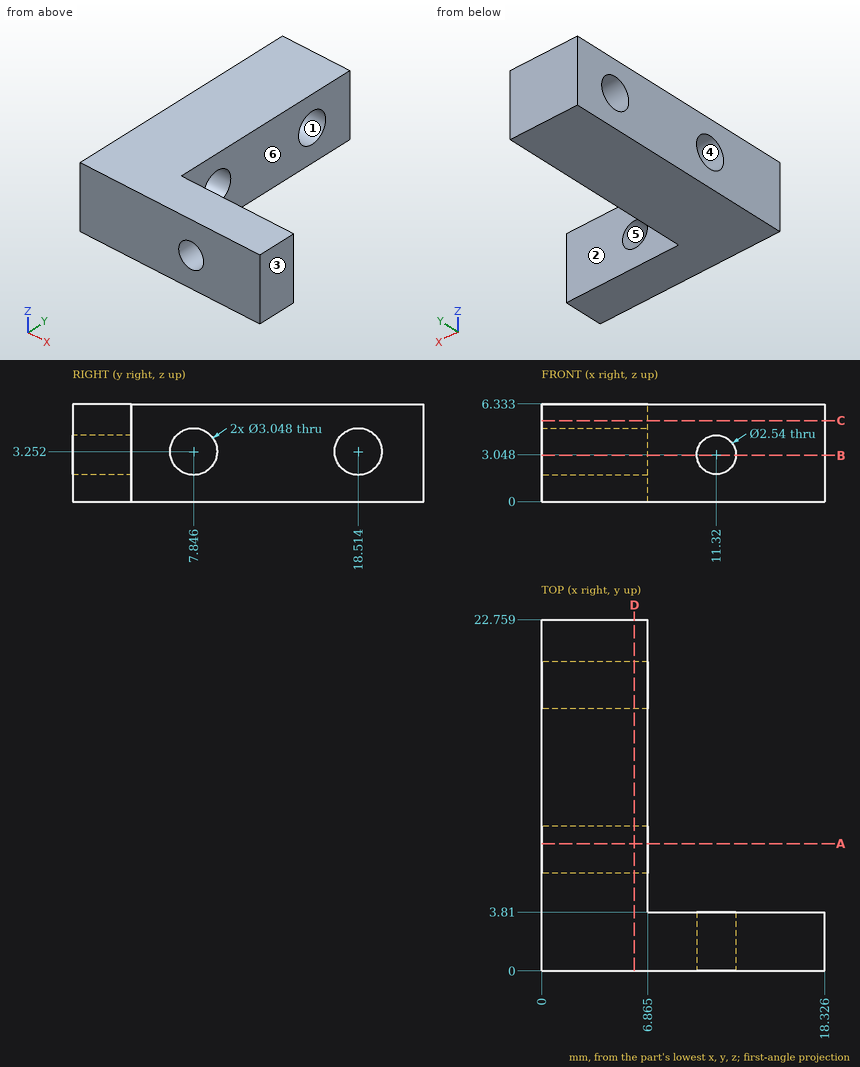
Drawing for the job (mm, zero at the part's lowest x, y, z). A direction names the side the tool comes from. Coordinates: 2 decimals unless noted, no trailing zeros. Write each loop counter-clockwise with the first axis right and the second up, starting at its lowest first coordinate (ties: lowest second). Pieces come first, ordered by that corner, then holes. Notation, with made-up numbers: (65.5, 21) -> (108.5, 21) arc R15 ccw to (108.5, 40) -> close; hole circle Ø9 at (46.5, -40). An arc over 180 degrees is marked (long way). One line per item, written item: value. Start each with the question number.
1) Slice it at C-C on z = 5.25. Write the cut outline in (x, y) (1 decimal).
2) Slice it at A-A on y = 8.25. Write the cut outline in (x, z) (1 decimal), then the cut area to 3 significant figures.
3) Slice it at D-D on x = 6. Write the cut outline in (y, z) (1 decimal).
4) Pull direction Y, two halves, no side cores. Call the marked faces 1, 2, 3 and 4: +Y half, -Y half, draft (parallel to the pull), parting line (faces both ways), or undercut.
5) Slice it at B-B on z = 3. Count the separate pieces of the cut face and the enclosed holes in it, then the cut area to 3 significant figures.
6) Probe probe 1 along Y at (x, z) = (2, 4.5) (1 decimal); probe 2 along Y at (x, z) = (1.5, 3); probe 3 along X at (y, z) = (16.25, 4) (1 decimal). List the from-to ranges inside material, lowest first.
7) Which spindle directions (+Z, -Z, +X, -X, +Y, -Y) get a long thin tool onto all of the face, cutting with end or side? Do the marked faces 5 and 6. Say none if no direction does.
8) Flat gauge pins, fed straight in: pin 1 Ø1.5 at (y, z) = (6.5, 2) entering from +X (1 decimal); pin 2 Ø1 at (x, z) = (16, 0.5) entering from +Y. Where does each tip first touch, or does it go through?
Answers follow:
1. outline: (0, 0) -> (18.3, 0) -> (18.3, 3.8) -> (6.9, 3.8) -> (6.9, 22.8) -> (0, 22.8) -> close
2. outline: (0, 0) -> (6.9, 0) -> (6.9, 1.8) -> (0, 1.8) -> close; (0, 4.7) -> (6.9, 4.7) -> (6.9, 6.3) -> (0, 6.3) -> close
2. area: 23.3 mm2
3. outline: (0, 0) -> (22.8, 0) -> (22.8, 6.3) -> (0, 6.3) -> close; hole circle Ø3 at (7.8, 3.3); hole circle Ø3 at (18.5, 3.3)
4. face 1: undercut
4. face 2: +Y half
4. face 3: draft
4. face 4: undercut
5. separate pieces: 4
5. enclosed holes: 0
5. area: 149 mm2
6. probe 1: 0 to 7, 8.7 to 17.6, 19.4 to 22.8
6. probe 2: 0 to 6.34, 9.35 to 17.01, 20.02 to 22.76
6. probe 3: 0 to 6.9
7. face 5: +Y, -Y
7. face 6: +Z, -Z, +X, +Y
8. pin 1: x = 6.9
8. pin 2: y = 3.81
